```python
from build123d import *

# Parameters (mm, degrees)
EXTRUDE_1_DEPTH        = 2
SKETCH_4_W             = 10
SKETCH_4_H             = 239
CUT_EXTRUDE_1640_DEPTH = 481.836770641
SKETCH_841_R           = 2.5
CUT_EXTRUDE_2_DEPTH    = 481.836770641
SKETCH_5_W             = 207
SKETCH_5_H             = 202
SKETCH_5_W_2           = 203
SKETCH_5_H_2           = 198
EXTRUDE_1_2_DEPTH      = 15
SKETCH_7_W             = 85
SKETCH_7_H             = 72
CUT_EXTRUDE_4_DEPTH    = 482.066523466
SKETCH_9_W             = 20.5
SKETCH_9_H             = 80
SKETCH_9_W_2           = 298
SKETCH_9_H_2           = 10.5
CUT_EXTRUDE_5_DEPTH    = 10
SKETCH_10_W            = 87
SKETCH_10_H            = 74
SKETCH_10_W_2          = 85
SKETCH_10_H_2          = 72
EXTRUDE_2_DEPTH        = 15


with BuildPart() as part:
    # 草图2 → Extrude 1 (new body)
    with BuildSketch(Plane(origin=(0, 0, 0), x_dir=(1, 0, 0), z_dir=(0, 1, 0))):
        Polygon((21, 21), (21, 0), (319, 0), (319, 21), (340, 21), (340, 319), (319, 319), (319, 340), (21, 340), (21, 319), (0, 319), (0, 21), align=None)
    extrude(amount=EXTRUDE_1_DEPTH)

    # 草图4 → Cut-Extrude 1640 (cut, through all)
    with BuildSketch(Plane(origin=(0, 2, 0), x_dir=(1, 0, 0), z_dir=(0, 1, 0))):
        with Locations((314.5, 170)):
            Rectangle(SKETCH_4_W, SKETCH_4_H)
    extrude(amount=-CUT_EXTRUDE_1640_DEPTH, mode=Mode.SUBTRACT)

    # Sketch 841 → 切除-拉伸2 (cut, through all)
    with BuildSketch(Plane(origin=(0, 2, 0), x_dir=(1, 0, 0), z_dir=(0, 1, 0))):
        with Locations(Location((10.5, 41, 0), (0, 0, 270))):
            Circle(SKETCH_841_R)
        with Locations(Location((10.5, 299, 0), (0, 0, 90))):
            Circle(SKETCH_841_R)
        with Locations(Location((329.5, 299, 0), (0, 0, 270))):
            Circle(SKETCH_841_R)
        with Locations(Location((329.5, 41, 0), (0, 0, 90))):
            Circle(SKETCH_841_R)
        with Locations(Location((41, 10.5, 0), (0, 0, 270))):
            Circle(SKETCH_841_R)
        with Locations(Location((299, 10.5, 0), (0, 0, 90))):
            Circle(SKETCH_841_R)
        with Locations(Location((299, 329.5, 0), (0, 0, 270))):
            Circle(SKETCH_841_R)
        with Locations(Location((41, 329.5, 0), (0, 0, 90))):
            Circle(SKETCH_841_R)
    extrude(amount=-CUT_EXTRUDE_2_DEPTH, mode=Mode.SUBTRACT)

    # 草图5 → Extrude 1 2 (add)
    with BuildSketch(Plane(origin=(0, 2, 0), x_dir=(1, 0, 0), z_dir=(0, 1, 0))):
        with Locations((142.5, 140)):
            Rectangle(SKETCH_5_W, SKETCH_5_H)
        with Locations((142.5, 140)):
            Rectangle(SKETCH_5_W_2, SKETCH_5_H_2, mode=Mode.SUBTRACT)
    extrude(amount=EXTRUDE_1_2_DEPTH)

    # 草图7 → 切除-拉伸4 (cut, through all)
    with BuildSketch(Plane(origin=(0, 2, 0), x_dir=(1, 0, 0), z_dir=(0, 1, 0))):
        with Locations((160, 278.5)):
            Rectangle(SKETCH_7_W, SKETCH_7_H)
    extrude(amount=-CUT_EXTRUDE_4_DEPTH, mode=Mode.SUBTRACT)

    # 草图9 → 切除-拉伸5 (cut)
    with BuildSketch(Plane(origin=(0, 2, 0), x_dir=(1, 0, 0), z_dir=(0, 1, 0))):
        with Locations((329.75, 136)):
            Rectangle(SKETCH_9_W, SKETCH_9_H)
        with Locations((170, 5.25)):
            Rectangle(SKETCH_9_W_2, SKETCH_9_H_2)
        with Locations((170, 334.75)):
            Rectangle(SKETCH_9_W_2, SKETCH_9_H_2)
    extrude(amount=-CUT_EXTRUDE_5_DEPTH, mode=Mode.SUBTRACT)

    # 草图10 → 拉伸-薄壁2 (add)
    with BuildSketch(Plane(origin=(0, 2, 0), x_dir=(1, 0, 0), z_dir=(0, 1, 0))):
        with Locations((160, 278.5)):
            Rectangle(SKETCH_10_W, SKETCH_10_H)
        with Locations((160, 278.5)):
            Rectangle(SKETCH_10_W_2, SKETCH_10_H_2, mode=Mode.SUBTRACT)
    extrude(amount=EXTRUDE_2_DEPTH)


solid = part.part
```
The model under review builds one solid part; all positions refer to its coordinate system, in mm. A direction names the side the tool comes from. Round coordinates to 2 decimals unless told otherwise and drop trailing zeros. Order: outer loops, then holes, each group sorted by start corner. A loop starts at its lowest first (then second) coordinate and runs counter-clockwise, first axis right, second up. Notation, with made-up numbers: (5.25, -33.5) -> (54.25, -33.5) arc R24 ccw to (54.25, -16.5) -> close; hole circle Ø2 at (72.25, 57). An arc over 180 degrees is marked (long way). Use a Markdown table: item, result.
Q1. Tool access review of faces 1 (the flat face through (141, 9, -41)), 2 (the flat face through (159, 9, -241.5)), 3 (the flat face through (159, 8, -314.5)), 4 (the flat face through (141, 9, -39)): name each direction out of +Z, -Z, +X, -X, +Y, -Y from which nothing blocks a thin tool from reaching the whole face with its end or side.
Values:
| item | result |
|---|---|
| face 1 | +Y |
| face 2 | +X, -X, +Y |
| face 3 | +Y, -Y |
| face 4 | +Z, +X, -X, +Y |
Q2. Clearance check with flat-ended pins moving along their axes: P1, Ø4, axis at x = 10.5, z = -299, coming from the +Y side; P2, Ø1, axis at y = 1, z = -17, coming from the -X side; P3, Ø3, axis at x = 216, z = -123.5, coming from the +Y side; P4, Ø4.5, axis at y = 12, z = -263, coming from the -X side. State where each tip first meets the part, or that it passes through.
Values:
| item | result |
|---|---|
| P1 | passes through |
| P2 | stops at x = 21 |
| P3 | stops at y = 2 |
| P4 | stops at x = 116.5 |
Q3. Mouldability with a two-part tool opening along X and no side actions: class faces 5 (the flat face through (39, 9, -139)), 6 (the flat face through (202.5, 8, -278)), 7 (the flat face through (141, 9, -241)) as +X half, -X half, draft (parallel to the pull), parting line (faces both ways), or undercut.
Values:
| item | result |
|---|---|
| face 5 | -X half |
| face 6 | undercut |
| face 7 | draft |
Q4. We need section C-C on x = 197. Write out the cut boundary in (y, z), then the cut area to 3 significant figures.
Values:
| item | result |
|---|---|
| outline | (0, -329.5) -> (2, -329.5) -> (2, -315.5) -> (17, -315.5) -> (17, -314.5) -> (0, -314.5) -> close; (0, -242.5) -> (17, -242.5) -> (17, -241.5) -> (2, -241.5) -> (2, -241) -> (17, -241) -> (17, -239) -> (2, -239) -> (2, -41) -> (17, -41) -> (17, -39) -> (2, -39) -> (2, -10.5) -> (0, -10.5) -> close |
| area | 584 mm^2 |
Q5. We need section D-D on z = -272. Write out the cut boundary in (x, y).
Values:
| item | result |
|---|---|
| outline | (0, 0) -> (117.5, 0) -> (117.5, 17) -> (116.5, 17) -> (116.5, 2) -> (0, 2) -> close; (202.5, 0) -> (309.5, 0) -> (309.5, 2) -> (203.5, 2) -> (203.5, 17) -> (202.5, 17) -> close; (319.5, 0) -> (340, 0) -> (340, 2) -> (319.5, 2) -> close |
Q6. For line 1 (X direction, y = 0.6, z = -41); line 2 (Z direction, x = 184.5, y = 5.75); line 3 (X direction, y = 1, z = -299), list the stretches that pass through material, from the lowest coordinate up.
Values:
| item | result |
|---|---|
| line 1 | x = 0 to 8, 13 to 327, 332 to 340 |
| line 2 | z = -315.5 to -314.5, -242.5 to -241.5, -241 to -239, -41 to -39 |
| line 3 | x = 0 to 8, 13 to 117.5, 202.5 to 327, 332 to 340 |
Q7. We need section B-B on z = -224. Write out the cut boundary in (x, y).
Values:
| item | result |
|---|---|
| outline | (0, 0) -> (309.5, 0) -> (309.5, 2) -> (246, 2) -> (246, 17) -> (244, 17) -> (244, 2) -> (41, 2) -> (41, 17) -> (39, 17) -> (39, 2) -> (0, 2) -> close; (319.5, 0) -> (340, 0) -> (340, 2) -> (319.5, 2) -> close |
Q8. We need section A-A on y = 10.25. Write out the cut boundary in (x, z).
Values:
| item | result |
|---|---|
| outline | (39, -241) -> (246, -241) -> (246, -39) -> (39, -39) -> close; (116.5, -315.5) -> (203.5, -315.5) -> (203.5, -241.5) -> (116.5, -241.5) -> close; hole (41, -239) -> (244, -239) -> (244, -41) -> (41, -41) -> close; hole (117.5, -314.5) -> (202.5, -314.5) -> (202.5, -242.5) -> (117.5, -242.5) -> close |
